Geometry check sheet. Reference: the model listing, model coordinates, mm. A direction names the side the tool comes from. Coordinates: 2 decimals unless noted, no trailing zeros. Write each loop counter-clockwise with the first axis right and the second up, starting at its lowest first coordinate (ties: lowest second). Pieces come first, ordered by that corner, then holes.
Autodesk Inventor part; units mm, degrees
ref_plane "YZ Plane" through (0, 0, 0) normal (1, 0, 0) x (0, 1, 0)
ref_plane "XZ Plane" through (0, 0, 0) normal (0, 1, 0) x (-1, 0, 0)
ref_plane "XY Plane" through (0, 0, 0) normal (0, 0, 1) x (1, 0, 0)
sketch "Sketch1" plane through (0, 0, 0) normal (0, 0, 1) x (1, 0, 0)
  circle A0 centre (0, 0) radius 4.7625
  circle A1 centre (0, 0) radius 3.1625
  dimension "d0" = 9.525
  dimension "d4" = 1.6
extrude "Extrusion1" add sketch "Sketch1" along normal blind 10
sketch "Sketch2" plane through (0, 0, 10) normal (0, 0, 1) x (1, 0, 0)
  circle A0 centre (0, 0) radius 14.5
  circle A1 centre (0, 0) radius 4.7625
  circle A2 centre (0, 0) radius 3.1625
  circle A3 centre (0, 0) radius 4.7625
  dimension "d5" = 29
extrude "Extrusion2" add sketch "Sketch2" along normal blind 5 contours A0 | A1
sketch "Sketch3" plane through (0, 0, 10) normal (0, 0, -1) x (-1, 0, 0)
  circle A0 centre (0, 0) radius 14.5
  circle A1 centre (0, 0) radius 12.9
  dimension "d8" = 1.6
extrude "Extrusion3" add sketch "Sketch3" along normal blind 5
fillet "Fillet1" radius 3 2 edges at (-3.1625, 0, 15) (-14.5, 0, 15)
properties part number "TA12" material "ABS Plastic"
1. Access from +Z, -Z, +X, -X, +Y, -Y to the whole of each face (thin tool, end or side, straight path). Record for faces 3 (the cylindrical face through (-1, 3, 6)), 4 (the cylindrical face through (2.796, 12.593, 7.535)).
Computed values:
face 3: +Z, -Z
face 4: -Z
2. Gauge pin test, flat ends, axial feed: pin 1 Ø6 at (x, z) = (3.5, 7.5) entering from -Y; pin 2 Ø6 at (x, z) = (8.5, 11.5) entering from -Y; pin 3 Ø2 at (x, z) = (7, 8) entering from -Y. Record the tip position at first contact, or that the pin passes through.
Computed values:
pin 1: stops at y = -14.49
pin 2: stops at y = -13.42
pin 3: stops at y = -13.2
3. Sectioned sample at C-C, the plane z = 7.5. Record the boundary of the cut face in (x, y) (1 decimal).
Computed values:
outline: circle Ø29 at (0, 0); circle Ø9.5 at (0, 0); hole circle Ø25.8 at (0, 0); hole circle Ø6.3 at (0, 0)
4. Thickness scan on line 1 along Y through (x, z) = (0, 6.6); line 2 along Z through (x, y) = (3.25, -5.5); line 3 along X through (y, z) = (-2, 2.75). Record the ranges inside material, lowest first.
Computed values:
line 1: y = -14.5 to -12.9, -4.76 to -3.16, 3.16 to 4.76, 12.9 to 14.5
line 2: z = 10 to 15
line 3: x = -4.32 to -2.45, 2.45 to 4.32
5. Draft check along Y on faces 1 (the flat face through (5, -5, 15)), 2 (the cylindrical face through (-3.78, 2.9, 4.93)). Enter one of: released by +Y, released by -Y, zero draft, split by the parting line, or undercut.
Computed values:
face 1: zero draft
face 2: undercut
6. Sectioned sample at A-A, the plane x = 0. Record the boundary of the cut face in (y, z), and give its area (3 significant figures).
Computed values:
outline: (-14.5, 5) - (-12.9, 5) - (-12.9, 10) - (-4.76, 10) - (-4.76, 0) - (-3.16, 0) - (-3.16, 12) arc R3 ccw to (-6.16, 15) - (-11.5, 15) arc R3 ccw to (-14.5, 12) - close; (3.16, 0) - (4.76, 0) - (4.76, 10) - (12.9, 10) - (12.9, 5) - (14.5, 5) - (14.5, 12) arc R3 ccw to (11.5, 15) - (6.16, 15) arc R3 ccw to (3.16, 12) - close
area: 154 mm2
7. Sectioned sample at D-D, the plane z = 4.5. Record the boundary of the cut face in (x, y) (1 decimal).
Computed values:
outline: circle Ø9.5 at (0, 0); hole circle Ø6.3 at (0, 0)
